```python
from build123d import *

# Parameters (mm, degrees)
SKETCH2_R           = 35
SKETCH2_R_2         = 27.5
BOSS_EXTRUDE2_DEPTH = 15
FILLET2_R           = 1
SKETCH4_R           = 27.5
SKETCH4_R_2         = 23.5
BOSS_EXTRUDE4_DEPTH = 14
BOSS_EXTRUDE5_DEPTH = 10
CIRPATTERN1_COUNT   = 5
FILLET3_R           = 4


with BuildPart() as part:
    # Sketch2 → Boss-Extrude2 (new, symmetric)
    with BuildSketch(Plane.XY):
        Circle(SKETCH2_R)
        Circle(SKETCH2_R_2, mode=Mode.SUBTRACT)
    extrude(amount=BOSS_EXTRUDE2_DEPTH, both=True)

    # Fillet2
    fillet2_edges = [part.edges().sort_by_distance(p)[0] for p in [
        (-35, 0, -15),
        (-35, 0, 15),
    ]]
    fillet(fillet2_edges, radius=FILLET2_R)

    # Sketch4 → Boss-Extrude4 (add, symmetric)
    with BuildSketch(Plane.XY):
        Circle(SKETCH4_R)
        Circle(SKETCH4_R_2, mode=Mode.SUBTRACT)
    extrude(amount=BOSS_EXTRUDE4_DEPTH, both=True)

    # Sketch5 → Boss-Extrude5 (add, symmetric)
    with BuildSketch(Plane.XY):
        with BuildLine():
            Line((-2.9938824, 23.308510638), (-4.5, 8.93028555))
            ThreePointArc((-4.5, 8.93028555), (0, -10), (4.5, 8.93028555))
            Line((4.5, 8.93028555), (2.9938824, 23.308510638))
            ThreePointArc((2.9938824, 23.308510638), (0, 23.5), (-2.9938824, 23.308510638))
        make_face()
    boss_extrude5 = extrude(amount=BOSS_EXTRUDE5_DEPTH, both=True)

    # CirPattern1: Boss-Extrude5 ×5 about axis
    cirpattern1_axis = Axis((0, 0, 0), (0, 0, 1))
    for i in range(1, CIRPATTERN1_COUNT):
        add(boss_extrude5.rotate(cirpattern1_axis, i * 360 / CIRPATTERN1_COUNT))

    # Fillet3
    # the kernel refuses this fillet: 4 mm, written as the material it adds along each edge
    with BuildSketch(Plane(origin=(-4.5, 8.93028555, 10), x_dir=(0.10417989743620854, 0.9945584693572224, 0), z_dir=(0, 0, -1)), Plane(origin=(-9.883782739, -1.520144324, 10), x_dir=(-0.9136879543386928, 0.40641643925458404, 0), z_dir=(0, 0, -1)), Plane(origin=(-1.60851367, -9.86978641, 10), x_dir=(-0.6688701083288824, -0.7433792963111827, 0), z_dir=(0, 0, -1)), Plane(origin=(8.88966662, -4.579719139, 10), x_dir=(0.5003034933326179, -0.8658501109078748, 0), z_dir=(0, 0, -1)), Plane(origin=(7.10262979, 7.039364323, 10), x_dir=(0.9780746718987476, 0.20825449860724982, 0), z_dir=(0, 0, -1))) as fillet3_piece_1:
        with BuildLine():
            CenterArc((1.956767483, -4), FILLET3_R, 90, 47.790159625)
            ThreePointArc((-1.005989395, -1.312608759), (-0.475813738, -0.677135992), (0, 0))
            Line((0, 0), (1.956767483, 0))
        make_face()
    extrude(amount=20)
    with BuildSketch(Plane(origin=(-7.10262979, 7.039364323, 10), x_dir=(-0.9780746718987477, 0.20825449860724976, 0), z_dir=(0, 0, -1)), Plane(origin=(-8.88966662, -4.579719139, 10), x_dir=(-0.5003034933326195, -0.8658501109078739, 0), z_dir=(0, 0, -1)), Plane(origin=(1.60851367, -9.86978641, 10), x_dir=(0.6688701083288834, -0.7433792963111817, 0), z_dir=(0, 0, -1)), Plane(origin=(9.883782739, -1.520144324, 10), x_dir=(0.9136879543386924, 0.4064164392545845, 0), z_dir=(0, 0, -1)), Plane(origin=(4.5, 8.93028555, 10), x_dir=(-0.10417989743620937, 0.9945584693572224, 0), z_dir=(0, 0, -1))) as fillet3_piece_2:
        with BuildLine():
            CenterArc((1.956767483, 4), FILLET3_R, 222.209840375, 47.790159625)
            ThreePointArc((-1.005989395, 1.312608759), (-0.475813738, 0.677135992), (0, 0))
            Line((0, 0), (1.956767483, 0))
        make_face()
    extrude(amount=20)


solid = part.part
```
Model file for the job. Use its own axes, mm. A direction names the side the tool comes from. Give positions to 0.01 mm unless a question says otherwise; leave off trailing zeros. Write each loop counter-clockwise with the first axis right and the second up, starting at its lowest first coordinate (ties: lowest second). Pieces come first, ordered by that corner, then holes. Notation, with made-up numbers: (5.5, 19) -> (20.5, 19) arc R29 ccw to (20.5, 51) -> close; hole circle Ø9 at (83.25, 18). An arc over 180 degrees is marked (long way). Use CSV: the item, a comma, the result in double quotes. Start each with the question number.
1) Drill centre lines: L1, parallel to Y at x = -20, z = -6.5; L2, parallel to Y at x = -17.5, z = -4.5; L3, parallel to X at y = 16.5, z = -4. Where is each one in solid material? Low to high.
2) Cut at C-C on y = 9. Count the separate pieces of the cut face and the enclosed holes in it, plus the area to 3 significant figures.
3) Tool access for faces 1 (the flat face through (20.2, 12.4, -14)), 2 (the cylindrical face through (-5.961, -26.846, 14.493)), 3 (the cylindrical face through (9.36, -4.74, 0.14)): list every direction of +Z, -Z, +X, -X, +Y, -Y with a clear straight run to the whole face (end or side of a thin tool).
4) Pin check, flat tips, straight feed: P1, Ø16.5, axis at x = 12.5, y = -4, coming from the +Z side; P2, Ø10, axis at y = 14, z = 11, coming from the -X side; P3, Ø4, axis at x = 3, z = -11, coming from the +Y side; P4, Ø8, axis at x = -13.5, y = 19.5, coming from the -Z side. Stop position of each tip, or through.
5) Cut at B-B on z = -12. List the corners of the cut face in (x, y), plus the area to 3 significant figures.
6) Two-plate mould, pull along X, no slides. Class faces 4 (the cylindrical face through (7.403, 7.436, 0.14)), 5 (the flat face through (7.039, -15.906, 0.14)), 6 (the flat face through (28, 0, 15)): released by +X, released by -X, zero draft, split by the parting line, or undercut.
7) Cut at A-A on z = 5. List the corners of the cut face in (x, y).
Final values:
1,L1,"y = -28.72 to -12.34, 2.98 to 9.79, 12.34 to 28.72"
1,L2,"y = -30.31 to -15.68, 1.87 to 9.25, 15.68 to 30.31"
1,L3,"x = -30.87 to -16.73, -3.71 to 3.71, 16.73 to 30.87"
2,separate pieces,"3"
2,enclosed holes,"0"
2,area,"1,120 mm2"
3,face 1,"-Z"
3,face 2,"+Z"
3,face 3,"+Z, -Z"
4,P1,"stops at z = 10"
4,P2,"stops at x = -33.82"
4,P3,"stops at y = 34.99"
4,P4,"stops at z = -15"
5,outline,"circle Ø70 at (0, 0); hole circle Ø47 at (0, 0)"
5,area,"2,110 mm2"
6,face 4,"undercut"
6,face 5,"undercut"
6,face 6,"zero draft"
7,outline,"circle Ø70 at (0, 0); hole (-23.09, 4.36) arc R23.5 ccw to (-16.12, -17.1) -> (-9.87, -6.27) arc R4 ccw to (-9.51, -3.09) arc R4 ccw to (-11.67, -0.72) -> close; hole (-21.24, 10.05) -> (-9.02, 7.45) arc R4 ccw to (-5.88, 8.09) arc R4 ccw to (-4.3, 10.88) -> (-2.99, 23.31) arc R23.5 ccw to start; hole (-11.28, -20.62) arc R23.5 ccw to (11.28, -20.62) -> (2.92, -11.32) arc R4 ccw to (0, -10) arc R4 ccw to (-2.92, -11.32) -> close; hole (2.99, 23.31) -> (4.3, 10.88) arc R4 ccw to (5.88, 8.09) arc R4 ccw to (9.02, 7.45) -> (21.24, 10.05) arc R23.5 ccw to start; hole (9.51, -3.09) arc R4 ccw to (9.87, -6.27) -> (16.12, -17.1) arc R23.5 ccw to (23.09, 4.36) -> (11.67, -0.72) arc R4 ccw to start"
